The model under review builds one solid part; all positions refer to its coordinate system, in mm. Face numbers are marked on the shaded views. Give positions to 0.01 mm unless a question says otherwise; leave off trailing zeros. Loops run counter-clockwise (first coordinate to the right, second up) from the corner with the lowest first, then second, coordinate; pieces in that order, holes last. Notation, with made-up numbers: M 32.25,-38.5 L 42.25,-38.5 A19 ccw 42.25,-15.5 Z; hole C -29.75,85 d1. An arc over 180 degrees is marked long. One line per item, written item: value. Start each with the question number.
Q1. For pin 1 (1.5 mm diameter, centred on y = 3.5, z = 3.5, fed in from -X) (3 decimals); pin 2 (5 mm diameter, centred on x = -30, y = -4, fed in from -Z); pin 3 (4 mm diameter, centred on x = 1, z = 4.5, fed in from -Y); pin 4 (0.7 mm diameter, centred on y = 0, z = 0, fed in from +X), all flat-tipped, find the tip position at first contact; note any pin that passes through.
Q2. Mouldability with a two-part tool opening along X and no side actions: class the marked faces 1, 2, 3 and 4 as released by +X, released by -X, zero draft, split by the parting line, or undercut.
Q3. To check wall thickness, follow line 1 along X through (y, z) = (2.75, -3.25) (3 decimals); line 2 along Y through (x, z) = (-42, 0); line 3 along X through (y, z) = (0.5, -4) (3 decimals). State the ranges of each line that lie inside material, in increasing order. Write a range as from..to.
Q4. We need section A-A on x = 42. Write out the cut boundary in (y, z) (3 decimals), plus the area to 3 significant figures.
```python
from build123d import *

# Parameters (mm, degrees)
SKETCH2_W          = 19
SKETCH2_H          = 14.6
SKETCH2_W_2        = 15
SKETCH2_H_2        = 10.6
CUT_EXTRUDE1_DEPTH = 2.8


with BuildPart() as part:
    # Sketch1 → Revolve1 (revolve)
    with BuildSketch(Plane(origin=(0, 0, 0), x_dir=(1, 0, 0), z_dir=(0, 1, 0))):
        Polygon((-49.285, 0.6), (-49.285, 1.95), (-42.185, 2.322095233), (-42.185, 4.1), (-45.685, 4.1), (-45.685, 5), (-38.835, 5), (-38.835, 4.74), (-31.985, 4.74), (-31.985, 3.885), (46.485, 3.885), (46.485, 6.805), (49.285, 6.805), (49.285, 0.75), (-31.985, 0.75), (-31.985, 0.6), align=None)
    revolve(axis=Axis((49.285, 0, 0), (-1, 0, 0)))

    # Sketch2 → Cut-Extrude1 (cut)
    with BuildSketch(Plane(origin=(49.285, 0, 0), x_dir=(0, 0, -1), z_dir=(1, 0, 0))):
        Rectangle(SKETCH2_W, SKETCH2_H)
        Rectangle(SKETCH2_W_2, SKETCH2_H_2, mode=Mode.SUBTRACT)
    extrude(amount=-CUT_EXTRUDE1_DEPTH, mode=Mode.SUBTRACT)


solid = part.part
```
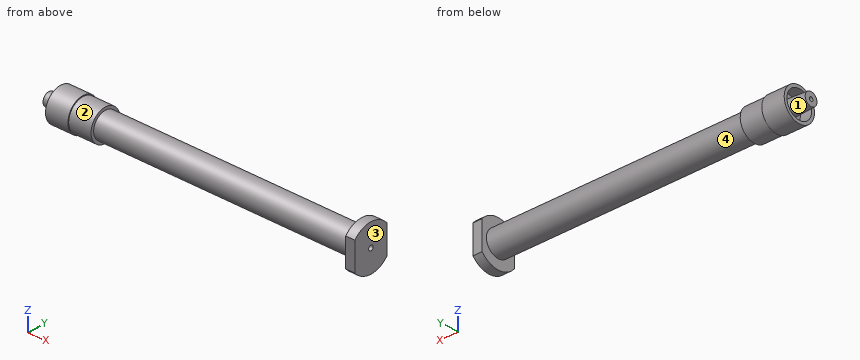
Solved:
1. pin 1: x = -45.685
1. pin 2: z = -4.04
1. pin 3: y = -2.97
1. pin 4: through
2. face 1: released by -X
2. face 2: undercut
2. face 3: released by +X
2. face 4: undercut
3. line 1: -45.685..-31.985, 46.485..49.285
3. line 2: -5..-0.6, 0.6..5
3. line 3: -42.185..-31.985, 46.485..49.285
4. outline: C 0,0 d7.77; hole C 0,0 d1.5
4. area: 45.6 mm2
